Part model, mm, in its own coordinate system. Face numbers are marked on the shaded views. A direction names the side the tool comes from. Round coordinates to 2 decimals unless told otherwise and drop trailing zeros. Loops run counter-clockwise (first coordinate to the right, second up) from the corner with the lowest first, then second, coordinate; pieces in that order, holes last.
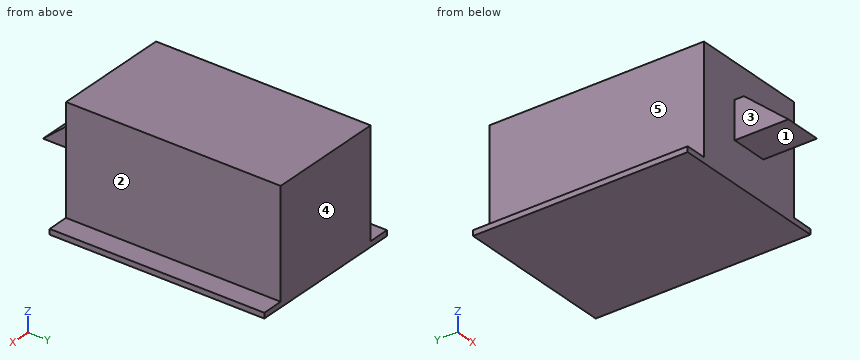
from build123d import *

# Parameters (mm, degrees)
F0_W     = 38.1
F0_H     = 50.8
F1_DEPTH = 1.27
F2_W     = 27.94
F2_H     = 50.8
F3_DEPTH = 25.4
F4_W     = 8.89
F4_H     = 8.89
F5_DEPTH = 12.7
F7_DEPTH = 8.89


with BuildPart() as f1:
    # F0 (on Top) → F1 (new body)
    with BuildSketch(Plane.XY):
        with Locations((-19.05, 25.4)):
            Rectangle(F0_W, F0_H)
    extrude(amount=F1_DEPTH)

    # F2 (on face) → F3 (join)
    with BuildSketch(Plane.XY.offset(1.27)):
        with Locations((-19.05, 25.4)):
            Rectangle(F2_W, F2_H)
    extrude(amount=F3_DEPTH)

    # F4 (on face) → F5 (join)
    with BuildSketch(Plane.XZ):
        with Locations((-19.05, 13.97)):
            Rectangle(F4_W, F4_H)
    extrude(amount=F5_DEPTH)

    # F6 (on face) → F7 (cut, through all)
    with BuildSketch(Plane(origin=(-23.495, 0, 0), x_dir=(0, -1, 0), z_dir=(-1, 0, 0))):
        Polygon((12.7, 18.415), (2.17834, 18.415), (12.7, 9.525), align=None)
    extrude(amount=-F7_DEPTH, mode=Mode.SUBTRACT)


solid = f1.part
1) Drop flat-ended pins along their axis: pin 1 Ø1.7 at (x, y) = (-18, -1.5) entering from +Z (3 decimals); pin 2 Ø5.5 at (x, y) = (-36.5, 21) entering from +Z; pin 3 Ø7.5 at (y, z) = (36.5, 11) entering from +X; pin 4 Ø2 at (x, y) = (-18, 32) entering from -Z. Give the stop position or say it passes through.
Values:
pin 1: stops at z = 18.415
pin 2: stops at z = 1.27
pin 3: stops at x = -5.08
pin 4: stops at z = 0
2) Wall check: line 1 along X through (y, z) = (5.5, 14.5); line 2 along Y through (x, z) = (-8, 12.5); line 3 along Z through (x, y) = (-37, 17.5). Give the ranges that are in metal, low to high.
Values:
line 1: x = -33.02 to -5.08
line 2: y = 0 to 50.8
line 3: z = 0 to 1.27
3) Slice it at B-B, the plane x = -20. Give the cut face in (y, z) (3 decimals), then the cut area to 3 significant figures.
Values:
outline: (-12.7, 9.525) - (0, 9.525) - (0, 0) - (50.8, 0) - (50.8, 26.67) - (0, 26.67) - (0, 18.415) - (-2.178, 18.415) - close
area: 1,420 mm2
4) Tool access for the marked faces 1, 2, 3, 4 and 5: list every direction of +Z, -Z, +X, -X, +Y, -Y with a clear straight run to the whole face (end or side of a thin tool).
Values:
face 1: -Z, +X, -X, -Y
face 2: +Z, +X, +Y, -Y
face 3: +Z, -Z, -X, -Y
face 4: +Z, -Z, +X, -X, +Y
face 5: +Z, -X, +Y, -Y
5) Slice it at D-D, the plane x = -27. Give the cut face in (y, z), then the cut area to 3 significant figures.
Values:
outline: (0, 0) - (50.8, 0) - (50.8, 26.67) - (0, 26.67) - close
area: 1,350 mm2
6) Slice it at C-C, the plane z = 8.25. Give the cut face in (x, y), then the cut area to 3 significant figures.
Values:
outline: (-33.02, 0) - (-5.08, 0) - (-5.08, 50.8) - (-33.02, 50.8) - close
area: 1,420 mm2
7) Slice it at A-A, the plane y = 17.5. Give the cut face in (x, z).
Values:
outline: (-38.1, 0) - (0, 0) - (0, 1.27) - (-5.08, 1.27) - (-5.08, 26.67) - (-33.02, 26.67) - (-33.02, 1.27) - (-38.1, 1.27) - close
